The model under review builds one solid part; all positions refer to its coordinate system, in mm. A direction names the side the tool comes from. Round coordinates to 2 decimals unless told otherwise and drop trailing zeros. Order: outer loops, then holes, each group sorted by start corner. A loop starts at its lowest first (then second) coordinate and runs counter-clockwise, first axis right, second up. Notation, with made-up numbers: (88.25, 20.25) - (101.25, 20.25) arc R15 ccw to (101.25, 25.25) - close; hole circle Ø2 at (60.5, 85.5). An arc over 180 degrees is marked (long way). One line per question, with ' | ' between items. Start each with the question number.
Item 1: Draft analysis for pull direction Y (two halves, no side actions). For faces 1 (the face through (22.5, -7, -14)), 2 (the face through (21, -31, -12)), 3 (the face through (-16, -23, -12.75)), state which applies: +Y half, -Y half, draft (parallel to the pull), parting line (faces both ways), or undercut.
Item 2: For L1, parallel to Y at x = 11.25, z = -11.5; L2, parallel to X at y = -17, z = -12.6; L3, parallel to X at y = 1.5, z = 10, list the stretches that pass through material, from the lowest coordinate up. Write a range as [from, to].
Item 3: Add section C-C on z = 6.75. State the section outline as (x, y) points.
Item 4: Add section A-A on z = 10. State the section outline as (x, y) points.
Item 5: Add section B-B on z = -9. State the section outline as (x, y) points, and give its area (3 significant figures).
Item 6: Insertion check: pin 1 Ø1.1 at (x, y) = (-21, -24) entering from -Z; pin 2 Ø1.5 at (x, y) = (15.5, -9) entering from +Z; pin 3 Ø0.8 at (x, y) = (21, -22) entering from -Z. Each pin has a flat end and moves straight along its axis. Give the tip position at first contact, or say it passes through.
Item 7: Tool access review of faces 4 (the face through (11.5, 1.5, -9.1)), 5 (the face through (-20, -23, -12.75)), 6 (the face through (0, -13.5, -15)): name each direction out of +Z, -Z, +X, -X, +Y, -Y from which nothing blocks a thin tool from reaching the whole face with its end or side.
from build123d import *

# Parameters (mm, degrees)
SKETCH1_W                      = 45
SKETCH1_H                      = 27
BOSS_EXTRUDE1_DEPTH            = 3
CUT_EXTRUDE1_REACH             = 28.41
SKETCH2_R                      = 1.75
SKETCH3_W                      = 45
SKETCH3_H                      = 35.5
BOSS_EXTRUDE2_DEPTH            = 3
SKETCH4_W                      = 45
SKETCH4_H                      = 22
BOSS_EXTRUDE3_DEPTH            = 3
SKETCH6_W                      = 45
SKETCH6_H                      = 19
CUT_EXTRUDE2_DEPTH             = 3
SKETCH7_W                      = 1
SKETCH7_H                      = 7
CUT_EXTRUDE3_DEPTH             = 1.5
SKETCH8_W                      = 45
SKETCH8_H                      = 7
CUT_EXTRUDE4_DEPTH             = 0.75
CUT_EXTRUDE5_REACH             = 49.87
SKETCH10_R                     = 2.25
CUT_EXTRUDE5_DIRECTION_2_DEPTH = 48.86961458
CHAMFER1_SIZE                  = 3


with BuildPart() as part:
    # Sketch1 → Boss-Extrude1 (new body)
    with BuildSketch(Plane(origin=(0, 0, 0), x_dir=(1, 0, 0), z_dir=(0, 1, 0))):
        Rectangle(SKETCH1_W, SKETCH1_H)
    extrude(amount=BOSS_EXTRUDE1_DEPTH)

    # Sketch2 → Cut-Extrude1 (cut, up to next)
    with BuildSketch(Plane(origin=(0, 3, 0), x_dir=(1, 0, 0), z_dir=(0, 1, 0)), mode=Mode.PRIVATE) as cut_extrude1_sk1:
        with Locations(Location((-10, 10, 0), (0, 0, 270))):
            Circle(SKETCH2_R)
    cut_extrude1_tool1 = extrude(cut_extrude1_sk1.sketch, amount=-CUT_EXTRUDE1_REACH, mode=Mode.PRIVATE) & part.part
    # Sketch2 → Cut-Extrude1 (cut, up to next)
    with BuildSketch(Plane(origin=(0, 3, 0), x_dir=(1, 0, 0), z_dir=(0, 1, 0)), mode=Mode.PRIVATE) as cut_extrude1_sk2:
        with Locations(Location((10, 10, 0), (0, 0, 270))):
            Circle(SKETCH2_R)
    cut_extrude1_tool2 = extrude(cut_extrude1_sk2.sketch, amount=-CUT_EXTRUDE1_REACH, mode=Mode.PRIVATE) & part.part
    # Sketch2 → Cut-Extrude1 (cut, up to next)
    with BuildSketch(Plane(origin=(0, 3, 0), x_dir=(1, 0, 0), z_dir=(0, 1, 0)), mode=Mode.PRIVATE) as cut_extrude1_sk3:
        with Locations(Location((10, -10, 0), (0, 0, 270))):
            Circle(SKETCH2_R)
    cut_extrude1_tool3 = extrude(cut_extrude1_sk3.sketch, amount=-CUT_EXTRUDE1_REACH, mode=Mode.PRIVATE) & part.part
    # Sketch2 → Cut-Extrude1 (cut, up to next)
    with BuildSketch(Plane(origin=(0, 3, 0), x_dir=(1, 0, 0), z_dir=(0, 1, 0)), mode=Mode.PRIVATE) as cut_extrude1_sk4:
        with Locations(Location((-10, -10, 0), (0, 0, 270))):
            Circle(SKETCH2_R)
    cut_extrude1_tool4 = extrude(cut_extrude1_sk4.sketch, amount=-CUT_EXTRUDE1_REACH, mode=Mode.PRIVATE) & part.part
    add(cut_extrude1_tool1.solids().sort_by_distance((-10, 3, -10))[0], mode=Mode.SUBTRACT)
    add(cut_extrude1_tool2.solids().sort_by_distance((10, 3, -10))[0], mode=Mode.SUBTRACT)
    add(cut_extrude1_tool3.solids().sort_by_distance((10, 3, 10))[0], mode=Mode.SUBTRACT)
    add(cut_extrude1_tool4.solids().sort_by_distance((-10, 3, 10))[0], mode=Mode.SUBTRACT)

    # Sketch3 → Boss-Extrude2 (add)
    with BuildSketch(Plane(origin=(0, 0, -13.5), x_dir=(-1, 0, 0), z_dir=(0, 0, -1))):
        with Locations((0, -14.75)):
            Rectangle(SKETCH3_W, SKETCH3_H)
    extrude(amount=BOSS_EXTRUDE2_DEPTH)

    # Sketch4 → Boss-Extrude3 (add)
    with BuildSketch(Plane.XY.offset(-13.5)):
        with Locations((0, -21.5)):
            Rectangle(SKETCH4_W, SKETCH4_H)
    extrude(amount=BOSS_EXTRUDE3_DEPTH)

    # Sketch6 → Cut-Extrude2 (cut)
    with BuildSketch(Plane(origin=(0, 0, -16.5), x_dir=(-1, 0, 0), z_dir=(0, 0, -1))):
        with Locations((0, -23)):
            Rectangle(SKETCH6_W, SKETCH6_H)
    extrude(amount=-CUT_EXTRUDE2_DEPTH, mode=Mode.SUBTRACT)

    # Sketch7 → Cut-Extrude3 (cut)
    with BuildSketch(Plane(origin=(0, 0, -13.5), x_dir=(-1, 0, 0), z_dir=(0, 0, -1))):
        with Locations((19, -23)):
            Rectangle(SKETCH7_W, SKETCH7_H)
        with Locations((21, -23)):
            Rectangle(SKETCH7_W, SKETCH7_H)
        with Locations((17, -23)):
            Rectangle(SKETCH7_W, SKETCH7_H)
        with Locations((15, -23)):
            Rectangle(SKETCH7_W, SKETCH7_H)
        with Locations((13, -23)):
            Rectangle(SKETCH7_W, SKETCH7_H)
        with Locations((11, -23)):
            Rectangle(SKETCH7_W, SKETCH7_H)
        with Locations((9, -23)):
            Rectangle(SKETCH7_W, SKETCH7_H)
        with Locations((7, -23)):
            Rectangle(SKETCH7_W, SKETCH7_H)
        with Locations((5, -23)):
            Rectangle(SKETCH7_W, SKETCH7_H)
        with Locations((3, -23)):
            Rectangle(SKETCH7_W, SKETCH7_H)
        with Locations((1, -23)):
            Rectangle(SKETCH7_W, SKETCH7_H)
        with Locations((-1, -23)):
            Rectangle(SKETCH7_W, SKETCH7_H)
        with Locations((-3, -23)):
            Rectangle(SKETCH7_W, SKETCH7_H)
        with Locations((-5, -23)):
            Rectangle(SKETCH7_W, SKETCH7_H)
        with Locations((-7, -23)):
            Rectangle(SKETCH7_W, SKETCH7_H)
        with Locations((-9, -23)):
            Rectangle(SKETCH7_W, SKETCH7_H)
        with Locations((-11, -23)):
            Rectangle(SKETCH7_W, SKETCH7_H)
        with Locations((-13, -23)):
            Rectangle(SKETCH7_W, SKETCH7_H)
        with Locations((-15, -23)):
            Rectangle(SKETCH7_W, SKETCH7_H)
        with Locations((-17, -23)):
            Rectangle(SKETCH7_W, SKETCH7_H)
        with Locations((-19, -23)):
            Rectangle(SKETCH7_W, SKETCH7_H)
        with Locations((-21, -23)):
            Rectangle(SKETCH7_W, SKETCH7_H)
    extrude(amount=-CUT_EXTRUDE3_DEPTH, mode=Mode.SUBTRACT)

    # Sketch8 → Cut-Extrude4 (cut)
    with BuildSketch(Plane(origin=(0, 0, -13.5), x_dir=(-1, 0, 0), z_dir=(0, 0, -1))):
        with Locations((0, -23)):
            Rectangle(SKETCH8_W, SKETCH8_H)
    extrude(amount=-CUT_EXTRUDE4_DEPTH, mode=Mode.SUBTRACT)

    # Sketch10 → Cut-Extrude5 (cut, up to next)
    with BuildSketch(Plane(origin=(0, 0, -13.5), x_dir=(-1, 0, 0), z_dir=(0, 0, -1)), mode=Mode.PRIVATE) as cut_extrude5_sk1:
        with Locations(Location((11.25, -29, 0), (0, 0, 180))):
            Circle(SKETCH10_R)
    cut_extrude5_tool1 = extrude(cut_extrude5_sk1.sketch, amount=-CUT_EXTRUDE5_REACH, mode=Mode.PRIVATE) & part.part
    # Sketch10 → Cut-Extrude5 (cut, up to next)
    with BuildSketch(Plane(origin=(0, 0, -13.5), x_dir=(-1, 0, 0), z_dir=(0, 0, -1)), mode=Mode.PRIVATE) as cut_extrude5_sk2:
        with Locations(Location((11.25, -17, 0), (0, 0, 180))):
            Circle(SKETCH10_R)
    cut_extrude5_tool2 = extrude(cut_extrude5_sk2.sketch, amount=-CUT_EXTRUDE5_REACH, mode=Mode.PRIVATE) & part.part
    # Sketch10 → Cut-Extrude5 (cut, up to next)
    with BuildSketch(Plane(origin=(0, 0, -13.5), x_dir=(-1, 0, 0), z_dir=(0, 0, -1)), mode=Mode.PRIVATE) as cut_extrude5_sk3:
        with Locations(Location((-11.25, -17, 0), (0, 0, 180))):
            Circle(SKETCH10_R)
    cut_extrude5_tool3 = extrude(cut_extrude5_sk3.sketch, amount=-CUT_EXTRUDE5_REACH, mode=Mode.PRIVATE) & part.part
    # Sketch10 → Cut-Extrude5 (cut, up to next)
    with BuildSketch(Plane(origin=(0, 0, -13.5), x_dir=(-1, 0, 0), z_dir=(0, 0, -1)), mode=Mode.PRIVATE) as cut_extrude5_sk4:
        with Locations(Location((-11.25, -29, 0), (0, 0, 180))):
            Circle(SKETCH10_R)
    cut_extrude5_tool4 = extrude(cut_extrude5_sk4.sketch, amount=-CUT_EXTRUDE5_REACH, mode=Mode.PRIVATE) & part.part
    add(cut_extrude5_tool1.solids().sort_by_distance((-11.25, -29, -13.5))[0], mode=Mode.SUBTRACT)
    add(cut_extrude5_tool2.solids().sort_by_distance((-11.25, -17, -13.5))[0], mode=Mode.SUBTRACT)
    add(cut_extrude5_tool3.solids().sort_by_distance((11.25, -17, -13.5))[0], mode=Mode.SUBTRACT)
    add(cut_extrude5_tool4.solids().sort_by_distance((11.25, -29, -13.5))[0], mode=Mode.SUBTRACT)

    # Sketch10 → Cut-Extrude5 direction 2 (cut)
    with BuildSketch(Plane(origin=(0, 0, -13.5), x_dir=(-1, 0, 0), z_dir=(0, 0, -1))):
        with Locations(Location((11.25, -29, 0), (0, 0, 180))):
            Circle(SKETCH10_R)
        with Locations(Location((11.25, -17, 0), (0, 0, 180))):
            Circle(SKETCH10_R)
        with Locations(Location((-11.25, -17, 0), (0, 0, 180))):
            Circle(SKETCH10_R)
        with Locations(Location((-11.25, -29, 0), (0, 0, 180))):
            Circle(SKETCH10_R)
    extrude(amount=CUT_EXTRUDE5_DIRECTION_2_DEPTH, mode=Mode.SUBTRACT)

    # Chamfer1
    chamfer1_edges = [part.edges().sort_by_distance(p)[0] for p in [
        (22.5, -10.5, -12),
        (-22.5, -10.5, -12),
        (22.5, -32.5, -12),
        (-22.5, -32.5, -12),
    ]]
    chamfer(chamfer1_edges, length=CHAMFER1_SIZE - 0.0001)  # a hair under: the kernel refuses the full size


solid = part.part
Determined:
1) face 1: draft | face 2: -Y half | face 3: undercut
2) L1: [-32.5, -31.25], [-26.75, -19.25], [-14.75, -10.5], [0, 3] | L2: [-22.5, -13.5], [-9, 9], [13.5, 22.5] | L3: [-22.5, -11.75], [-8.25, 8.25], [11.75, 22.5]
3) outline: (-22.5, 0) - (22.5, 0) - (22.5, 3) - (-22.5, 3) - close
4) outline: (-22.5, 0) - (-11.75, 0) - (-11.75, 3) - (-22.5, 3) - close; (-8.25, 0) - (8.25, 0) - (8.25, 3) - (-8.25, 3) - close; (11.75, 0) - (22.5, 0) - (22.5, 3) - (11.75, 3) - close
5) outline: (-22.5, 0) - (-11.44, 0) - (-11.44, 3) - (-22.5, 3) - close; (-8.56, 0) - (8.56, 0) - (8.56, 3) - (-8.56, 3) - close; (11.44, 0) - (22.5, 0) - (22.5, 3) - (11.44, 3) - close | area: 118 mm2
6) pin 1: z = -12.75 | pin 2: z = -13.5 | pin 3: z = -12
7) face 4: +Y | face 5: -Z, +X, -X | face 6: -Z, +X, -X, -Y
